Geometry: final body of the model. Coordinates: model frame, mm. Round coordinates to 2 decimals unless told otherwise and drop trailing zeros. Loops run counter-clockwise (first coordinate to the right, second up) from the corner with the lowest first, then second, coordinate; pieces in that order, holes last. Notation, with made-up numbers: M 83,13.5 L 125,13.5 A20 cw 125,20.5 Z; hole C 79.25,33.25 d10. An arc over 180 degrees is marked long. Answer as a JSON object with one key per item and string values.
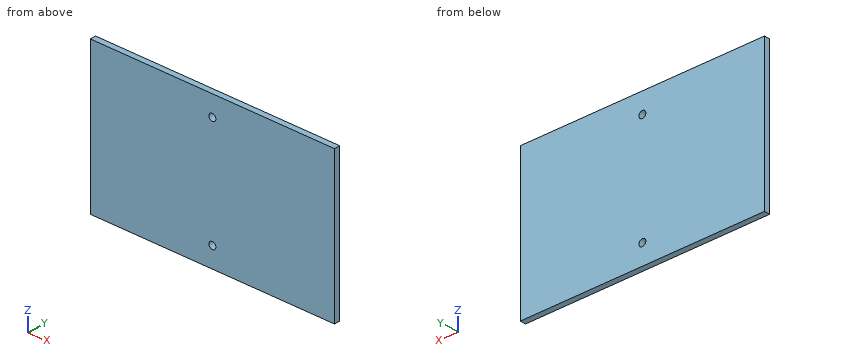
```python
from build123d import *

# Parameters (mm, degrees)
SKETCH1_W           = 210
SKETCH1_H           = 120
BOSS_EXTRUDE1_DEPTH = 5
SKETCH3_R           = 3
CUT_EXTRUDE1_DEPTH  = 10
SKETCH4_W           = 210
SKETCH4_H           = 5
BOSS_EXTRUDE2_DEPTH = 5
SKETCH5_W           = 210
SKETCH5_H           = 5
BOSS_EXTRUDE3_DEPTH = 5


with BuildPart() as part:
    # Sketch1 → Boss-Extrude1 (new body)
    with BuildSketch(Plane(origin=(0, 0, 0), x_dir=(1, 0, 0), z_dir=(0, 1, 0))):
        Rectangle(SKETCH1_W, SKETCH1_H)
    extrude(amount=BOSS_EXTRUDE1_DEPTH)

    # Sketch3 → Cut-Extrude1 (cut)
    with BuildSketch(Plane(origin=(0, 5, 0), x_dir=(1, 0, 0), z_dir=(0, 1, 0))):
        with Locations(Location((0, 47.5, 0), (0, 0, 270))):
            Circle(SKETCH3_R)
        with Locations(Location((0, -47.5, 0), (0, 0, 270))):
            Circle(SKETCH3_R)
    extrude(amount=-CUT_EXTRUDE1_DEPTH, mode=Mode.SUBTRACT)

    # Sketch4 → Boss-Extrude2 (add)
    with BuildSketch(Plane.XY.offset(60)):
        with Locations((0, 2.5)):
            Rectangle(SKETCH4_W, SKETCH4_H)
    extrude(amount=BOSS_EXTRUDE2_DEPTH)

    # Sketch5 → Boss-Extrude3 (add)
    with BuildSketch(Plane(origin=(0, 0, -60), x_dir=(-1, 0, 0), z_dir=(0, 0, -1))):
        with Locations((0, 2.5)):
            Rectangle(SKETCH5_W, SKETCH5_H)
    extrude(amount=BOSS_EXTRUDE3_DEPTH)


solid = part.part
```
1) Cut plane B-B on z = 47.5. Return the cut outline in (x, y), and give its area (3 significant figures).
Geometry results:
{"outline": "M -105,0 L -3,0 L -3,5 L -105,5 Z; M 3,0 L 105,0 L 105,5 L 3,5 Z", "area": "1,020 mm2"}
2) Line query: probe 1 along X at (y, z) = (1.5, 47.5). Output: solid intervals per line, ascending.
Geometry results:
{"probe 1": "-105 to -3, 3 to 105"}
3) Cut plane A-A on x = 0. Return the cut outline in (y, z), and give its area (3 significant figures).
Geometry results:
{"outline": "M 0,-65 L 5,-65 L 5,-50.5 L 0,-50.5 Z; M 0,-44.5 L 5,-44.5 L 5,44.5 L 0,44.5 Z; M 0,50.5 L 5,50.5 L 5,65 L 0,65 Z", "area": "590 mm2"}
